Input: part model. Units: mm. Frame: model coordinates. A direction names the side the tool comes from. Coordinates: 2 decimals unless noted, no trailing zeros. Write each loop counter-clockwise with the first axis right and the second up, starting at its lowest first coordinate (ties: lowest second). Pieces come first, ordered by that corner, then holes.
1) Section query B-B (x = 70). Output: boundary loops of the cut face in (y, z), then the cut area to 3 significant figures.
2) Section query A-A (z = -41). Output: boundary loops of the cut face in (x, y).
3) Draft query along X for faces 1 (the cylindrical face through (53.685, 1.201, -15.21)), 2 (the cylindrical face through (74.16, -1.72, -12.33)), 3 (the flat face through (39, 0, -55)), 4 (the flat face through (79, 8, -27)). Return one class per face: pulls with the +X half, pulls with the -X half, needs draft (parallel to the pull), parting line crosses it, or undercut.
4) Line query: L1, parallel to Z at x = 55, y = -6; L2, parallel to Z at x = 25, y = -5.25; L3, parallel to Y at x = 70, z = -15. Output: solid intervals per line, ascending.
5) Section query C-C (y = -8.5). Output: boundary loops of the cut face in (x, z), then the cut area to 3 significant figures.
6) Section query D-D (z = -31.5). Output: boundary loops of the cut face in (x, y), then the cut area to 3 significant figures.
7) Set-up query: faces 5 (the flat face through (70, -5, -25)), 6 (the cylindrical face through (30.7, -2.4, -15.2)), 7 (the flat face through (39, 0, 0)). Return all of +Z, -Z, +X, -X, +Y, -Y with unobstructed straight access to the full face (end or side cutting, diameter ignored); none if empty.
8) Pin query (flat end, axial travel): pin 1 Ø16.5 at (x, z) = (55, -41) entering from +Y. Return the tip coordinate at first contact, or that it passes through.
from build123d import *

# Parameters (mm, degrees)
SKETCH1_W                                           = 80
SKETCH1_H                                           = 55
BOSS_EXTRUDE1_DEPTH                                 = 10
M12_TAPPED_HOLE1_D                                  = 10.2
M16X1_5_TAPPED_HOLE1_D                              = 14.5
CBORE_FOR_M8_HEX_SOCKET_HEAD_CAP_SCREW2_D           = 9
CBORE_FOR_M8_HEX_SOCKET_HEAD_CAP_SCREW2_CBORE_D     = 14
CBORE_FOR_M8_HEX_SOCKET_HEAD_CAP_SCREW2_CBORE_DEPTH = 30
F_8_0_8_DIAMETER_HOLE1_D                            = 8
F_8_0_8_DIAMETER_HOLE1_DEPTH                        = 30
F_8_0_8_DIAMETER_HOLE1_TIP                          = 2.403442476
CHAMFER1_SIZE                                       = 3


with BuildPart() as part:
    # Sketch1 → Boss-Extrude1 (new, symmetric)
    with BuildSketch(Plane(origin=(0, 0, 0), x_dir=(1, 0, 0), z_dir=(0, 1, 0))):
        with Locations((40, 27.5)):
            Rectangle(SKETCH1_W, SKETCH1_H)
    extrude(amount=BOSS_EXTRUDE1_DEPTH, both=True)

    # M12 Tapped Hole1 (through all)
    with Locations(Plane(origin=(0, 10, 0), x_dir=(1, 0, 0), z_dir=(0, 1, 0))):
        with Locations((25, 41)):
            Hole(M12_TAPPED_HOLE1_D / 2)

    # M16x1.5 Tapped Hole1 (through all)
    with Locations(Plane(origin=(0, 10, 0), x_dir=(1, 0, 0), z_dir=(0, 1, 0))):
        with Locations((55, 41)):
            Hole(M16X1_5_TAPPED_HOLE1_D / 2)

    # CBORE for M8 Hex Socket Head Cap Screw2 (through all)
    with Locations(Plane(origin=(0, 0, -55), x_dir=(-1, 0, 0), z_dir=(0, 0, -1))):
        with Locations((-70, 0), (-10, 0)):
            CounterBoreHole(CBORE_FOR_M8_HEX_SOCKET_HEAD_CAP_SCREW2_D / 2, CBORE_FOR_M8_HEX_SOCKET_HEAD_CAP_SCREW2_CBORE_D / 2, CBORE_FOR_M8_HEX_SOCKET_HEAD_CAP_SCREW2_CBORE_DEPTH)

    # Ø8.0 (8) Diameter Hole1
    with Locations(Plane.XY):
        with Locations((27.5, 0), (57.5, 0)):
            Hole(F_8_0_8_DIAMETER_HOLE1_D / 2, depth=F_8_0_8_DIAMETER_HOLE1_DEPTH)
            with Locations((0, 0, -(F_8_0_8_DIAMETER_HOLE1_DEPTH + F_8_0_8_DIAMETER_HOLE1_TIP / 2))):  # 118° drill point
                Cone(0, F_8_0_8_DIAMETER_HOLE1_D / 2, F_8_0_8_DIAMETER_HOLE1_TIP, mode=Mode.SUBTRACT)

    # Chamfer1
    chamfer1_edges = [part.edges().sort_by_distance(p)[0] for p in [
        (80, 10, -27.5),
        (0, 10, -27.5),
        (80, -10, -27.5),
        (0, -10, -27.5),
    ]]
    chamfer(chamfer1_edges, length=CHAMFER1_SIZE)


solid = part.part
Answer:
1. outline: (-10, -55) - (-7, -55) - (-7, -25) - (-4.5, -25) - (-4.5, 0) - (-10, 0) - close; (4.5, -25) - (7, -25) - (7, -55) - (10, -55) - (10, 0) - (4.5, 0) - close
1. area: 455 mm2
2. outline: (0, -7) - (3, -10) - (19.9, -10) - (19.9, 10) - (3, 10) - (0, 7) - close; (30.1, -10) - (47.75, -10) - (47.75, 10) - (30.1, 10) - close; (62.25, -10) - (77, -10) - (80, -7) - (80, 7) - (77, 10) - (62.25, 10) - close; hole circle Ø14 at (10, 0); hole circle Ø14 at (70, 0)
3. face 1: undercut
3. face 2: undercut
3. face 3: needs draft
3. face 4: pulls with the +X half
4. L1: z = -55 to -48.25, -33.75 to 0
4. L2: z = -55 to -46.1, -35.9 to 0
4. L3: y = -10 to -4.5, 4.5 to 10
5. outline: (1.5, -55) - (78.5, -55) - (78.5, 0) - (1.5, 0) - close; hole circle Ø10.2 at (25, -41); hole circle Ø14.5 at (55, -41)
5. area: 3,990 mm2
6. outline: (0, -7) - (3, -10) - (77, -10) - (80, -7) - (80, 7) - (77, 10) - (3, 10) - (0, 7) - close; hole circle Ø14 at (10, 0); hole circle Ø3.01 at (27.5, 0); hole circle Ø3.01 at (57.5, 0); hole circle Ø14 at (70, 0)
6. area: 1,260 mm2
7. face 5: -Z
7. face 6: +Z
7. face 7: +Z, +X, -X, +Y, -Y
8. pin 1: stops at y = 10
